from build123d import *

# Parameters (mm, degrees)
ESQUISSE1_R                  = 1.65
BOSS_EXTRU_1_DEPTH           = 20
ENL_V_MAT_EXTRU_3_DEPTH      = 20
ENL_V_MAT_EXTRU_3_DEPTH_BACK = 20
ESQUISSE2_W                  = 10.952034034
ESQUISSE2_H                  = 5
CONG_1_R                     = 3
D_GAGEMENT_M41_D             = 4
D_GAGEMENT_M41_DEPTH         = 10
D_GAGEMENT_M41_CSINK_D       = 6
D_GAGEMENT_M41_CSINK_ANGLE   = 90
D_GAGEMENT_M41_TIP           = 1.201721238


with BuildPart() as part:
    # Esquisse1 → Boss.-Extru.1 (new body)
    with BuildSketch(Plane.XY):
        with BuildLine():
            Line((30, -1.65), (2.323790008, -1.65))
            ThreePointArc((2.323790008, -1.65), (-1.307669683, 2.532291452), (0, -2.85))
            Line((0, -2.85), (30, -2.85))
            Line((30, -2.85), (30, -1.65))
        make_face()
        Circle(ESQUISSE1_R, mode=Mode.SUBTRACT)
    extrude(amount=BOSS_EXTRU_1_DEPTH)

    # Esquisse2 → Enlèv. mat.-Extru.3 (cut, two sides: drawn at the far end of the back side and taken through both)
    with BuildSketch(Plane(origin=(0, -1.65, 0), x_dir=(1, 0, 0), z_dir=(0, 1, 0)).offset(-ENL_V_MAT_EXTRU_3_DEPTH_BACK)):
        with Locations((-2.176017017, -2.5)):
            Rectangle(ESQUISSE2_W, ESQUISSE2_H)
        with Locations((-2.176017017, -12.5)):
            Rectangle(ESQUISSE2_W, ESQUISSE2_H)
    extrude(amount=ENL_V_MAT_EXTRU_3_DEPTH + ENL_V_MAT_EXTRU_3_DEPTH_BACK, mode=Mode.SUBTRACT)

    # Congé1
    cong_1_edges = [part.edges().sort_by_distance(p)[0] for p in [
        (30, -2.25, 20),
        (30, -2.25, 0),
    ]]
    fillet(cong_1_edges, radius=CONG_1_R)

    # Dégagement M41
    with Locations(Plane(origin=(0, -1.65, 0), x_dir=(1, 0, 0), z_dir=(0, 1, 0))):
        with Locations((11.75, -14.25), (22.25, -6.75)):
            CounterSinkHole(D_GAGEMENT_M41_D / 2, D_GAGEMENT_M41_CSINK_D / 2, depth=D_GAGEMENT_M41_DEPTH, counter_sink_angle=D_GAGEMENT_M41_CSINK_ANGLE)
            with Locations((0, 0, -(D_GAGEMENT_M41_DEPTH + D_GAGEMENT_M41_TIP / 2))):  # 118° drill point
                Cone(0, D_GAGEMENT_M41_D / 2, D_GAGEMENT_M41_TIP, mode=Mode.SUBTRACT)


solid = part.part
Design review of the part built by this model. Coordinates are the model's own, in mm. A direction names the side the tool comes from. Coordinates: 2 decimals unless noted, no trailing zeros. Order: outer loops, then holes, each group sorted by start corner. A loop starts at its lowest first (then second) coordinate and runs counter-clockwise, first axis right, second up. Notation, with made-up numbers: (28, -19.75) - (41, -19.75) arc R31 cw to (41, 16.25) - close; hole circle Ø9 at (69, -29). An arc over 180 degrees is marked (long way). Put each result on its own line as item: value.
1) Take a section at C-C, the plane x = 22.25. Give the boundary of the cut face in (y, z).
Response values:
outline: (-2.85, 0) - (-1.65, 0) - (-1.65, 3.75) - (-2.65, 4.75) - (-2.85, 4.75) - close; (-2.85, 8.75) - (-2.65, 8.75) - (-1.65, 9.75) - (-1.65, 20) - (-2.85, 20) - close
2) Take a section at A-A, the plane y = 0. Give the boundary of the cut face in (x, z).
Response values:
outline: (-2.85, 5) - (-1.65, 5) - (-1.65, 10) - (-2.85, 10) - close; (-2.85, 15) - (-1.65, 15) - (-1.65, 20) - (-2.85, 20) - close; (1.65, 5) - (2.85, 5) - (2.85, 10) - (1.65, 10) - close; (1.65, 15) - (2.85, 15) - (2.85, 20) - (1.65, 20) - close
3) The part is to be moulded in two halves that separate along Y. For faces 1 (the face through (2, -1, 10)), 2 (the face through (-1.216, 1.115, 17.465)), say which applies: released by +Y, released by -Y, zero draft, split by the parting line, or undercut.
Response values:
face 1: zero draft
face 2: undercut
4) Tool access review of faces 3 (the face through (3.3, -2, 13)), 4 (the face through (3.3, -2, 3)), 5 (the face through (29.1, -2.24, 19.14)): name each direction out of +Z, -Z, +X, -X, +Y, -Y from which nothing blocks a thin tool from reaching the whole face with its end or side.
Response values:
face 3: -X, +Y, -Y
face 4: -Z, -X, +Y, -Y
face 5: +Z, +X, +Y, -Y
5) Take a section at D-D, the plane z = 14.25. Give the boundary of the cut face in (x, y).
Response values:
outline: (3.3, -2.85) - (9.75, -2.85) - (9.75, -2.65) - (8.75, -1.65) - (3.3, -1.65) - close; (13.75, -2.85) - (30, -2.85) - (30, -1.65) - (14.75, -1.65) - (13.75, -2.65) - close
6) Wall thickness on L1, parallel to Z at x = 11.75, y = -2.7; L2, parallel to X at y = -2.8, z = 14.25; L3, parallel to Z at x = 22.25, y = -2.8: over which ranges is each line inside the solid? List them lowest first. Write a range as from..to.
Response values:
L1: z = 0..12.25, 16.25..20
L2: x = 3.3..9.75, 13.75..30
L3: z = 0..4.75, 8.75..20
7) Insertion check: P1, Ø2.5, axis at x = 22.25, z = 6.75, coming from the +Y side; P2, Ø4, axis at x = 23.5, z = 6, coming from the +Y side; P3, Ø3, axis at y = -1.5, z = 7, coming from the -X side; P4, Ø1.3, axis at y = -2.5, z = 3.5, coming from the -X side. Each pin has a flat end and moves straight along its axis. Give the tip position at first contact, or say it passes through.
Response values:
P1: passes through
P2: stops at y = -1.65
P3: stops at x = -2.85
P4: stops at x = 3.3
8) Take a section at B-B, the plane z = 6.75. Give the boundary of the cut face in (x, y), and give its area (3 significant figures).
Response values:
outline: (0, -2.85) - (20.25, -2.85) - (20.25, -2.65) - (19.25, -1.65) - (2.32, -1.65) arc R2.85 ccw (long way) to start; (24.25, -2.85) - (30, -2.85) - (30, -1.65) - (25.25, -1.65) - (24.25, -2.65) - close; hole circle Ø3.3 at (0, 0)
area: 45.2 mm²
